Here's how the part is built. I have some questions about the finished solid (model axes, mm). A direction names the side the tool comes from. Round coordinates to 2 decimals unless told otherwise and drop trailing zeros. Write each loop counter-clockwise with the first axis right and the second up, starting at its lowest first coordinate (ties: lowest second). Pieces come first, ordered by that corner, then holes. Notation, with made-up numbers: M 60,51 L 90,51 A23 ccw 90,73 Z; hole C 43,52 d2. An arc over 180 degrees is marked long. Write item = value, one per line. Start each with the question number.
(1) I need wall thicknesses on line 1 along X through (y, z) = (22, -1); line 2 along Z through (x, y) = (176.5, 17.5); line 3 along X through (y, z) = (11, -8.25). Which ranges of each line are inside material? Lowest first, please.
(2) If we mould it in two halves opening along X, with no side actions, what happens to faces 4 (the flat face through (248, 24.843, 0)), 5 (the flat face through (199.822, 19, -6)), 6 (the flat face through (223.952, 19, -6)), 7 (the flat face through (214.74, 28.9, -3.25))? For each: released by +X, released by -X, zero draft, split by the parting line, or undercut.
(3) Will these pins go through, and if not, where does the flat tip stop? pin 1 Ø0.6 at (x, z) = (187, 0) entering from +Y; pin 2 Ø6 at (y, z) = (26, -7.5) entering from +X; pin 3 Ø11.5 at (x, y) = (254, 14.5) entering from -Z; pin 4 Ø5.5 at (x, y) = (269.04, 17.48) entering from +Z.
(4) On a 3-axis mill with a long thin cutter (end or side, diameter ignored), from which of +Z, -Z, +X, -X, +Y, -Y can I reach the whole of each face in a straight line? I mean faces 1 (the flat face through (212, 6, -0.586)), 2 (the flat face through (174, 16, -0.586)), 3 (the flat face through (201.822, 21, 0)). Say none if no direction works.
(5) I want a section at A-A (x = 176). List the corners of the cut face in (y, z) for me.
```python
from build123d import *

# Parameters (mm, degrees)
SKETCH_W             = 24.13
SKETCH_H             = 24.13
SKETCH_R             = 3.3782
PAD_DEPTH            = 2
PAD001_DEPTH         = 12.065
SKETCH002_R          = 6.35
POCKET_DEPTH         = 22.7167864376
PAD002_DEPTH         = 2
SKETCH004_R          = 2.4
PAD003_DEPTH         = 2
POCKET001_DEPTH      = 2.54
FILLET_R             = 0.508
BODY_PLACEMENT_ANGLE = 315
SKETCH010_R          = 2.4
PAD007_DEPTH         = 2
PAD008_DEPTH         = 2.032
PAD009_DEPTH         = 2.032


with BuildPart() as part:
    # Sketch → Pad (new body)
    with BuildSketch(Plane.XY):
        with Locations((0, 12.065)):
            Rectangle(SKETCH_W, SKETCH_H)
        with Locations((0, 12.065)):
            Circle(SKETCH_R, mode=Mode.SUBTRACT)
    extrude(amount=PAD_DEPTH)

    # Sketch001 → Pad001 (join, symmetric)
    with BuildSketch(Plane.YZ):
        with BuildLine():
            Line((0, 2), (22.7157864376, 24.7157864376))
            Line((22.7157864376, 24.7157864376), (24.13, 23.3015728753))
            Line((24.13, 23.3015728753), (4.5355339059, 3.7071067812))
            ThreePointArc((4.5355339059, 3.7071067812), (4.3187611546, 2.6173165676), (5.2426406871, 2))
            Line((5.2426406871, 2), (0, 2))
        make_face()
    extrude(amount=PAD001_DEPTH, both=True)

    # Sketch002 (on Face7 of Pad001) → Pocket (cut, through all)
    with BuildSketch(Plane.XY.offset(2)):
        with Locations((0, 12.065)):
            Circle(SKETCH002_R)
    extrude(amount=POCKET_DEPTH, mode=Mode.SUBTRACT)

    # Sketch003 (on Face9 of Pocket) → Pad002 (join)
    with BuildSketch(Plane.YZ.offset(12.065)):
        with BuildLine():
            ThreePointArc((17.8909137548, 17.06248663), (15.9782409773, 7.4468312404), (24.13, 2))
            Line((2.8284271247, 2), (24.13, 2))
            Line((17.8909137548, 17.06248663), (2.8284271247, 2))
        make_face()
    pad002 = extrude(amount=-PAD002_DEPTH)

    # Mirrored: Pad002 across YZ
    add(pad002.mirror(Plane.YZ))

    # Sketch004 (on Face5 of Mirrored) → Pad003 (join)
    with BuildSketch(Plane(origin=(0, -1, 1), x_dir=(1, 0, 0), z_dir=(0, -0.7071067812, 0.7071067812))):
        Polygon((-12.065, 33.5391868224), (-25.4, 24.8427001924), (-25.4, 10.1107001924), (-12.065, 1.4142135624), align=None)
        with Locations((-19.05, 17.4767001924)):
            Circle(SKETCH004_R, mode=Mode.SUBTRACT)
    pad003 = extrude(amount=-PAD003_DEPTH)

    # Mirrored001: Pad003 across Sketch004 V_Axis
    add(pad003.mirror(Plane(origin=(0, -1, 1), x_dir=(0, -0.7071067812, 0.7071067812), z_dir=(1, 0, 0))))

    # Sketch006 (on Face5 of Mirrored001) → Pocket001 (cut)
    with BuildSketch(Plane(origin=(0, -1, 1), x_dir=(1, 0, 0), z_dir=(0, -0.7071067812, 0.7071067812))):
        with BuildLine():
            Line((25.4, 24.8427001924), (25.4, 33.5391868224))
            Line((25.4, 33.5391868224), (-25.4, 33.5391868224))
            Line((-25.4, 33.5391868224), (-25.4, 24.8427001924))
            Line((-25.4, 24.8427001924), (-10.065, 24.8427001924))
            Line((-10.065, 16.2914440713), (-10.065, 24.8427001924))
            ThreePointArc((-10.065, 16.2914440713), (0, 6.2264440713), (10.065, 16.2914440713))
            Line((10.065, 16.2914440713), (10.065, 24.8427001924))
            Line((10.065, 24.8427001924), (25.4, 24.8427001924))
        make_face()
    extrude(amount=-POCKET001_DEPTH, mode=Mode.SUBTRACT)

    # Fillet
    fillet_edges = [part.edges().sort_by_distance(p)[0] for p in [
        (-25.4, 17.273549, 17.859335),
        (25.4, 17.273549, 17.859335),
    ]]
    fillet(fillet_edges, radius=FILLET_R)


with BuildPart() as part_1:
    # Body placement: moved
    add(part.part.rotate(Axis((0, 0, 0), (1, 0, 0)), BODY_PLACEMENT_ANGLE))

    # Sketch010 (on Face11 of Clone) → Pad007 (new body)
    with BuildSketch(Plane.XY.offset(1.4142135624)):
        with BuildLine():
            Line((-24.892, 24.8427001924), (-62.992, 24.8427001924))
            ThreePointArc((-62.992, 24.8427001924), (-63.3512102448, 24.6939104372), (-63.5, 24.3347001924))
            Line((-63.5, 24.3347001924), (-63.5, 10.6187001924))
            ThreePointArc((-63.5, 10.6187001924), (-63.3512102448, 10.2594899476), (-62.992, 10.1107001924))
            Line((-62.992, 10.1107001924), (-24.892, 10.1107001924))
            Line((-24.892, 10.1107001924), (-24.892, 24.8427001924))
        make_face()
        with Locations((-57.15, 17.4767001924)):
            Circle(SKETCH010_R, mode=Mode.SUBTRACT)
    pad007 = extrude(amount=-PAD007_DEPTH)

    # Mirrored003: Pad007 across Sketch010 V_Axis
    add(pad007.mirror(Plane(origin=(0, 0, 1.4142135624), x_dir=(0, 0, 1), z_dir=(1, 0, 0))))

    # Sketch011 (on Face21 of Mirrored003) → Pad008 (join)
    with BuildSketch(Plane(origin=(0, 17.5114994361, -17.5114994361), x_dir=(-1, 0, 0), z_dir=(0, 0.7071067812, -0.7071067812))):
        with BuildLine():
            Line((12.065, 0), (12.065, 22.86))
            ThreePointArc((12.065, 22.86), (11.6930256121, 23.7580256121), (10.795, 24.13))
            Line((10.795, 24.13), (-10.795, 24.13))
            ThreePointArc((-10.795, 24.13), (-11.6930256121, 23.7580256121), (-12.065, 22.86))
            Line((-12.065, 22.86), (-12.065, 0))
            Line((12.065, 0), (-12.065, 0))
        make_face()
        with BuildLine():
            ThreePointArc((3.3782, 15.6718), (0, 19.05), (-3.3782, 15.6718))
            Line((-3.3782, 15.6718), (-3.3782, 9.7282))
            ThreePointArc((-3.3782, 9.7282), (0, 6.35), (3.3782, 9.7282))
            Line((3.3782, 15.6718), (3.3782, 9.7282))
        make_face(mode=Mode.SUBTRACT)
    extrude(amount=-PAD008_DEPTH)

    # Sketch012 (on Face13 of Pad008) → Pad009 (join)
    with BuildSketch(Plane(origin=(-12.065, 0, 0), x_dir=(0, -0.7071067812, 0.7071067812), z_dir=(-1, 0, 0))):
        Polygon((-24.13, 2), (-2.8284271247, 2), (-24.13, 23.3015728753), align=None)
    pad009 = extrude(amount=-PAD009_DEPTH)

    # Mirrored004: Pad009 across YZ
    add(pad009.mirror(Plane.YZ))


with BuildPart() as part_2:
    # Body002 placement: moved
    add(part_1.part.moved(Location((211.8868, 0, 0))))


solid = part_2.part
```
Returned:
q1.line_1 = 199.82 to 201.85, 221.92 to 223.95
q1.line_2 = -0.59 to 1.41
q1.line_3 = 199.82 to 208.88, 214.89 to 223.95
q2.face_4 = zero draft
q2.face_5 = released by -X
q2.face_6 = released by +X
q2.face_7 = undercut
q3.pin_1 = 24.84
q3.pin_2 = 223.95
q3.pin_3 = -0.59
q3.pin_4 = 1.41
q4.face_1 = none
q4.face_2 = -Z, -X, +Y, -Y
q4.face_3 = +Z
q5.outline = M 10.11,-0.59 L 24.84,-0.59 L 24.84,1.41 L 10.11,1.41 Z
